The listing builds one solid part. Answer for the finished solid, in the listing's coordinates (mm). Give positions to 0.01 mm unless a question says otherwise; leave off trailing zeros. Loops run counter-clockwise (first coordinate to the right, second up) from the corner with the lowest first, then second, coordinate; pieces in that order, holes last.
Item 1: Section D-D, the plane x = 0 is taken. Give the vertices of the cut face in (y, z).
Item 2: Each of these flat-tipped pins is pushed along its axis until it touches: pin 1 Ø1 at (x, z) = (38, 1.5) entering from +Y; pin 2 Ø1.5 at (y, z) = (-36.5, 1.5) entering from -X; pin 3 Ø1.5 at (y, z) = (-54, 1.5) entering from +X. Where does it stop, or does it pass through?
Item 3: Section A-A, the plane z = 1.75 is taken. Give the vertices of the cut face in (x, y).
Item 4: Section B-B, the plane x = 28 is taken. Give the vertices of the cut face in (y, z), and give its area (3 significant figures).
Item 5: Section C-C, the plane y = -24.5 is taken. Give the vertices of the cut face in (x, z), and give its area (3 significant figures).
Item 6: Consider line 1 along X through (y, z) = (-57, 1.55); line 2 along Y through (x, z) = (-1, 3.2); line 3 along Y through (x, z) = (-3, 3.8). Determine where each line is inside the solid, lowest interval first.
from build123d import *

# Parameters (mm, degrees)
SKETCH_1_R          = 9.53
SKETCH_1_R_2        = 5.03
EXTRUDE_1_DEPTH     = 4
CUT_EXTRUDE_1_DEPTH = 10


with BuildPart() as part:
    # 草图1 → 凸台-拉伸1 (new body)
    with BuildSketch(Plane.XY):
        with BuildLine():
            Line((-60.484665535, -44.140957036), (-17.492328922, -1.148620423))
            ThreePointArc((-17.492328922, -1.148620423), (-0.984866816, 17.502312343), (17.510762826, 0.821026949))
            Line((17.510762826, 0.821026949), (60.595126742, -44.176306244))
            ThreePointArc((60.595126742, -44.176306244), (69.43811394, -58.606931767), (56.568542495, -69.598542495))
            Line((56.568542495, -69.598542495), (-56.568542495, -69.598542495))
            ThreePointArc((-56.568542495, -69.598542495), (-69.447058297, -58.549635813), (-60.484665535, -44.140957036))
        make_face()
        Circle(SKETCH_1_R, mode=Mode.SUBTRACT)
        with Locations((-56.568542495, -56.568542495)):
            Circle(SKETCH_1_R_2, mode=Mode.SUBTRACT)
        with Locations((56.568542495, -56.568542495)):
            Circle(SKETCH_1_R_2, mode=Mode.SUBTRACT)
    extrude(amount=EXTRUDE_1_DEPTH)

    # 草图2 → 切除-拉伸1 (cut)
    with BuildSketch(Plane.XY.offset(4)):
        with BuildLine():
            Line((-35.944637397, -47.236581954), (-6.146065042, -19.193110209))
            ThreePointArc((-6.146065042, -19.193110209), (-1.455267075, -17.291512681), (3.291241318, -19.049442373))
            Line((3.291241318, -19.049442373), (35.061663803, -47.175010024))
            ThreePointArc((35.061663803, -47.175010024), (35.878352511, -50.484569716), (33.073110812, -52.421264017))
            Line((33.073110812, -52.421264017), (-33.888630519, -52.421264017))
            ThreePointArc((-33.888630519, -52.421264017), (-36.677361968, -50.527146879), (-35.944637397, -47.236581954))
        make_face()
    extrude(amount=-CUT_EXTRUDE_1_DEPTH, mode=Mode.SUBTRACT)


solid = part.part
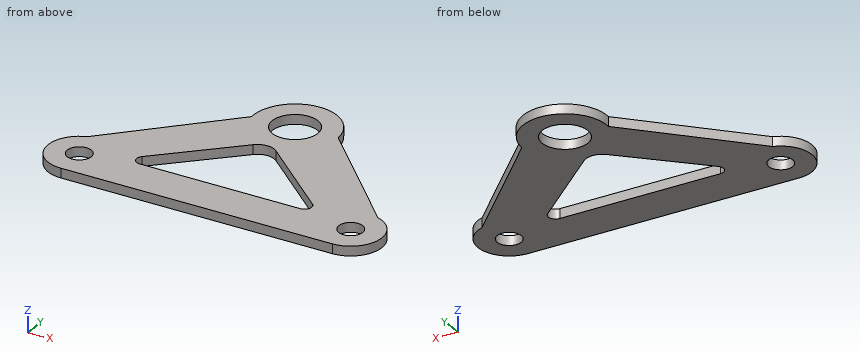
Worked answers:
1. outline: (-69.6, 0) - (-52.42, 0) - (-52.42, 4) - (-69.6, 4) - close; (-17.42, 0) - (-9.53, 0) - (-9.53, 4) - (-17.42, 4) - close; (9.53, 0) - (17.53, 0) - (17.53, 4) - (9.53, 4) - close
2. pin 1: stops at y = -20.06
2. pin 2: stops at x = -53.59
2. pin 3: stops at x = 69.47
3. outline: (-60.48, -44.14) arc R13.03 ccw to (-56.57, -69.6) - (56.57, -69.6) arc R13.03 ccw to (60.6, -44.18) - (17.51, 0.82) arc R17.53 ccw (long way) to (-17.49, -1.15) - close; hole circle Ø10.06 at (-56.57, -56.57); hole (-35.94, -47.24) arc R3 ccw to (-33.89, -52.42) - (33.07, -52.42) arc R3 ccw to (35.06, -47.18) - (3.29, -19.05) arc R7 ccw to (-6.15, -19.19) - close; hole circle Ø19.06 at (0, 0); hole circle Ø10.06 at (56.57, -56.57)
4. outline: (-69.6, 0) - (-52.42, 0) - (-52.42, 4) - (-69.6, 4) - close; (-40.92, 0) - (-10.13, 0) - (-10.13, 4) - (-40.92, 4) - close
4. area: 192 mm2
5. outline: (-40.84, 0) - (-11.79, 0) - (-11.79, 4) - (-40.84, 4) - close; (9.45, 0) - (41.76, 0) - (41.76, 4) - (9.45, 4) - close
5. area: 245 mm2
6. line 1: x = -69.59 to -61.58, -51.56 to 51.56, 61.58 to 69.59
6. line 2: y = -69.6 to -52.42, -17.3 to -9.48, 9.48 to 17.5
6. line 3: y = -69.6 to -52.42, -17.49 to -9.05, 9.05 to 17.27
